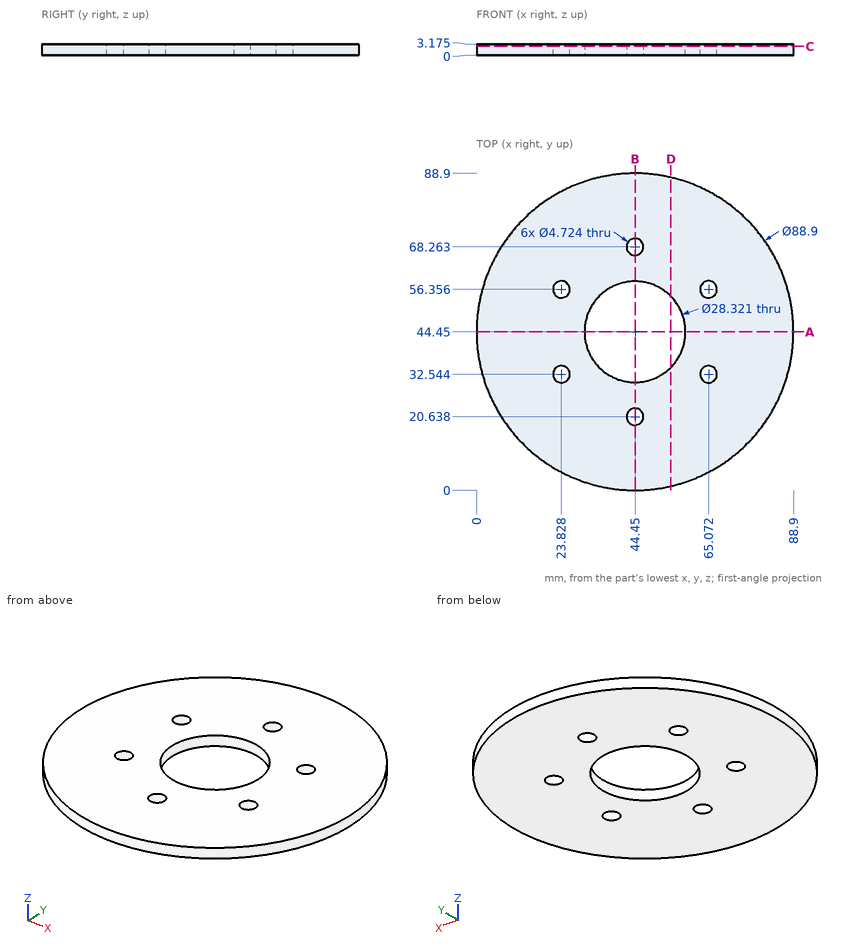
Geometry: see drawing. Coordinates: mm, zero at the bounding-box minimum. Give positions to 0.01 mm unless a question says otherwise; leave off trailing zeros. Write each loop counter-clockwise with the first axis right and the second up, starting at its lowest first coordinate (ties: lowest second). Pieces come first, ordered by that corner, then holes. Notation, with made-up numbers: M 75,-32 L 86,-32 A11 ccw 86,-25 Z; hole C 2,-21 d8. An arc over 180 degrees is marked long. Return JSON: item names as keys, results as strings. Group by question number.
1) First-contact query: pin 1 Ø3 at (x, y) = (65.07, 56.36) entering from -Z; pin 2 Ø1.5 at (x, z) = (68, 2.5) entering from +Y. Flat tips, straight axial feed; report the tip coordinate or a pass-through.
2) Cut plane A-A, the plane y = 44.45. Output: boundary loops of the cut face in (x, z) (1 decimal).
3) Cut plane D-D, the plane x = 54.5. Output: boundary loops of the cut face in (y, z) (1 decimal).
4) Cut plane C-C, the plane z = 2.5. Give the number of separate pieces and of enclosed holes in the cut face, then the cut area to 3 significant figures.
5) Cut plane B-B, the plane x = 44.45. Output: boundary loops of the cut face in (y, z) (1 decimal).
6) Ray query, L1, parallel to X at y = 56.5, z = 2.3 (1 decimal); L2, parallel to X at y = 46.5, z = 3.05; L3, parallel to Y at x = 39, z = 0.3 (1 decimal). Return the intervals inside material, ascending.
Data:
{
 "1": {"pin 1": "passes through", "pin 2": "stops at y = 82.61"},
 "2": {"outline": "M 0,0 L 30.3,0 L 30.3,3.2 L 0,3.2 Z; M 58.6,0 L 88.9,0 L 88.9,3.2 L 58.6,3.2 Z"},
 "3": {"outline": "M 1.2,0 L 34.5,0 L 34.5,3.2 L 1.2,3.2 Z; M 54.4,0 L 87.7,0 L 87.7,3.2 L 54.4,3.2 Z"},
 "4": {"separate pieces": "1", "enclosed holes": "7", "area": "5,470 mm²"},
 "5": {"outline": "M 0,0 L 18.3,0 L 18.3,3.2 L 0,3.2 Z; M 23,0 L 30.3,0 L 30.3,3.2 L 23,3.2 Z; M 58.6,0 L 65.9,0 L 65.9,3.2 L 58.6,3.2 Z; M 70.6,0 L 88.9,0 L 88.9,3.2 L 70.6,3.2 Z"},
 "6": {"L1": "x = 1.7 to 21.5, 26.2 to 37, 51.9 to 62.7, 67.4 to 87.2", "L2": "x = 0.05 to 30.44, 58.46 to 88.85", "L3": "y = 0.3 to 31.4, 57.5 to 88.6"}
}
